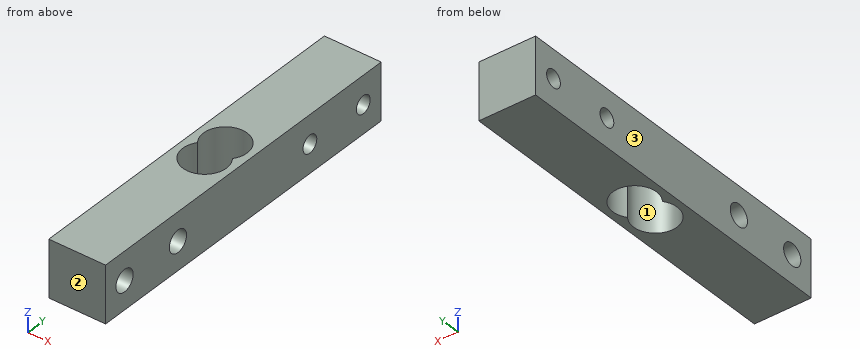
```python
from build123d import *

# Parameters (mm, degrees)
SKETCH1_W           = 13
SKETCH1_H           = 13
BOSS_EXTRUDE1_DEPTH = 80
CUT_EXTRUDE1_DEPTH  = 13
SKETCH3_R           = 2
SKETCH3_R_2         = 2.5
CUT_EXTRUDE2_DEPTH  = 13


with BuildPart() as part:
    # Sketch1 → Boss-Extrude1 (new body)
    with BuildSketch(Plane(origin=(0, 0, 0), x_dir=(1, 0, 0), z_dir=(0, 1, 0))):
        Rectangle(SKETCH1_W, SKETCH1_H)
    extrude(amount=BOSS_EXTRUDE1_DEPTH)

    # Sketch2 → Cut-Extrude1 (cut)
    with BuildSketch(Plane.XY.offset(6.5)):
        with BuildLine():
            ThreePointArc((-4, 40), (0, 32), (4, 40))
            ThreePointArc((4, 40), (0, 48), (-4, 40))
        make_face()
    extrude(amount=-CUT_EXTRUDE1_DEPTH, mode=Mode.SUBTRACT)

    # Sketch3 → Cut-Extrude2 (cut)
    with BuildSketch(Plane(origin=(6.5, 0, 0), x_dir=(0, 0, -1), z_dir=(1, 0, 0))):
        with Locations((0, 74.8)):
            Circle(SKETCH3_R)
        with Locations((0, 59.3)):
            Circle(SKETCH3_R)
        with Locations((0, 21)):
            Circle(SKETCH3_R_2)
        with Locations((0, 5.5)):
            Circle(SKETCH3_R_2)
    extrude(amount=-CUT_EXTRUDE2_DEPTH, mode=Mode.SUBTRACT)


solid = part.part
```
Model file for the job. Use its own axes, mm. Face numbers are marked on the shaded views. Coordinates: 2 decimals unless noted, no trailing zeros. Loops run counter-clockwise (first coordinate to the right, second up) from the corner with the lowest first, then second, coordinate; pieces in that order, holes last. Notation, with made-up numbers: M 15,7 L 47,7 A12 ccw 47,12 Z; hole C 68.25,53 d6. An arc over 180 degrees is marked long. Use CSV: the item, a comma, the result in double quotes. Start each with the question number.
1. Band-saw the part on B-B, the plane x = -3. List the corners of the cut face in (y, z).
2. Band-saw the part on D-D, the plane y = 74.8. List the corners of the cut face in (x, z).
3. Band-saw the part on C-C, the plane z = 0.5. List the corners of the cut face in (x, y).
4. Flat gauge pin, fed straight in: pin 1 (3.5 mm diameter, centred on y = 59.3, z = 0, fed in from -X). Where does the tip first touch, or does it go through?
5. Band-saw the part on A-A, the plane y = 21. List the corners of the cut face in (x, z).
6. Probe probe 1 along Y at (x, z) = (0.25, 0); probe 2 along Y at (x, z) = (2.25, 0); probe 3 along Y at (x, z) = (5.75, -1.25). List the from-to ranges inside material, lowest first. Write a range as [from, to].
7. Two-plate mould, pull along X, no slides. Class the marked faces 1, 2 and 3: pulls with the +X half, pulls with the -X half, needs draft (parallel to the pull), parting line crosses it, or undercut.
Entries:
1,outline,"M 0,-6.5 L 33,-6.5 L 33,6.5 L 0,6.5 Z; M 47,-6.5 L 80,-6.5 L 80,6.5 L 47,6.5 Z; hole C 5.5,0 d5; hole C 21,0 d5; hole C 59.3,0 d4; hole C 74.8,0 d4"
2,outline,"M -6.5,-6.5 L 6.5,-6.5 L 6.5,-2 L -6.5,-2 Z; M -6.5,2 L 6.5,2 L 6.5,6.5 L -6.5,6.5 Z"
3,outline,"M -6.5,0 L 6.5,0 L 6.5,3.05 L -6.5,3.05 Z; M -6.5,7.95 L 6.5,7.95 L 6.5,18.55 L -6.5,18.55 Z; M -6.5,23.45 L 6.5,23.45 L 6.5,57.36 L -6.5,57.36 Z; M -6.5,61.24 L 6.5,61.24 L 6.5,72.86 L -6.5,72.86 Z; M -6.5,76.74 L 6.5,76.74 L 6.5,80 L -6.5,80 Z; hole M -4,40 A5 ccw long 4,40 A5 ccw long Z"
4,pin 1,"passes through"
5,outline,"M -6.5,-6.5 L 6.5,-6.5 L 6.5,-2.5 L -6.5,-2.5 Z; M -6.5,2.5 L 6.5,2.5 L 6.5,6.5 L -6.5,6.5 Z"
6,probe 1,"y = [0, 3], [8, 18.5], [23.5, 32.01], [47.99, 57.3], [61.3, 72.8], [76.8, 80]"
6,probe 2,"y = [0, 3], [8, 18.5], [23.5, 32.53], [47.47, 57.3], [61.3, 72.8], [76.8, 80]"
6,probe 3,"y = [0, 3.33], [7.67, 18.83], [23.17, 57.74], [60.86, 73.24], [76.36, 80]"
7,face 1,"undercut"
7,face 2,"needs draft"
7,face 3,"pulls with the -X half"
